from build123d import *

# Parameters (mm, degrees)
SKETCH1_W           = 70
SKETCH1_H           = 30
BOSS_EXTRUDE1_DEPTH = 10
SKETCH2_R           = 6
CUT_EXTRUDE1_DEPTH  = 6
SKETCH3_R           = 3.2
CUT_EXTRUDE2_DEPTH  = 77.393717019
SKETCH9_R           = 14.8
BOSS_EXTRUDE3_DEPTH = 6.3


with BuildPart() as part:
    # Sketch1 → Boss-Extrude1 (new body)
    with BuildSketch(Plane.XY):
        with Locations((35, -15)):
            Rectangle(SKETCH1_W, SKETCH1_H)
    extrude(amount=BOSS_EXTRUDE1_DEPTH)

    # Sketch2 → Cut-Extrude1 (cut)
    with BuildSketch(Plane.XY.offset(10)):
        with Locations((10, -15)):
            Circle(SKETCH2_R)
        with Locations((60, -15)):
            Circle(SKETCH2_R)
    extrude(amount=-CUT_EXTRUDE1_DEPTH, mode=Mode.SUBTRACT)

    # Sketch3 → Cut-Extrude2 (cut, through all)
    with BuildSketch(Plane.XY.offset(4)):
        with Locations((10, -15)):
            Circle(SKETCH3_R)
        with Locations((60, -15)):
            Circle(SKETCH3_R)
    extrude(amount=-CUT_EXTRUDE2_DEPTH, mode=Mode.SUBTRACT)

    # Sketch9 → Boss-Extrude3 (add)
    with BuildSketch(Plane(origin=(0, 0, 0), x_dir=(1, 0, 0), z_dir=(0, 1, 0))):
        with Locations((35, -25.4)):
            Circle(SKETCH9_R)
        with BuildLine():
            Line((49.8, -25.4), (49.8, -10))
            Line((49.8, -10), (20.2, -10))
            Line((20.2, -10), (20.2, -25.4))
            ThreePointArc((20.2, -25.4), (35, -10.6), (49.8, -25.4))
        make_face()
    extrude(amount=-BOSS_EXTRUDE3_DEPTH)


solid = part.part
Work out the finished part from the listing and answer in its coordinate system (mm). A direction names the side the tool comes from. Round coordinates to 2 decimals unless told otherwise and drop trailing zeros. Write each loop counter-clockwise with the first axis right and the second up, starting at its lowest first coordinate (ties: lowest second). Pieces come first, ordered by that corner, then holes. Notation, with made-up numbers: (50, 42) -> (92, 42) arc R30 ccw to (92, 67) -> close; hole circle Ø3 at (40, 60.5). An arc over 180 degrees is marked (long way). Answer as CSV lines item,"result". Start each with the question number.
(1) The part is cut by section D-D, the plane y = -10.75. Give the vertices of the cut face in (x, z), then the cut area to 3 significant figures.
(2) The mould has two halves that part along Y. Classify faces 4 (the cylindrical face through (9.22, -9.05, 7.04)), 5 (the flat face through (20.2, -3, 18)), 6 (the flat face through (35, -6.3, 25)): +Y half, -Y half, draft (parallel to the pull), parting line (faces both ways), or undercut.
(3) Each of these flat-tipped pins is pushed along its axis until it touches: pin 1 (11 mm diameter, centred on x = 60, y = -15, fed in from +Z); pin 2 (10 mm diameter, centred on x = 12, z = 30.5, fed in from -Y); pin 3 (4 mm diameter, centred on x = 52.5, y = -3.5, fed in from +Z); pin 4 (7 mm diameter, centred on y = -4.5, z = 19.5, fed in from +X). Where does it stop, or does it pass through?
(4) Find the intervals of material crossed by probe 1 along Y at (x, z) = (10, 2); probe 2 along Y at (x, z) = (10, 5.55); probe 3 along Z at (x, y) = (18, -3), in increasing order.
(5) The part is cut by section C-C, the plane z = 5. Give the vertices of the cut face in (x, y), then the cut area to 3 significant figures.
(6) A tool of negligible diameter and unlimited length cuts with its end or side. For faces 1 (the flat face through (49.8, -3, 18)), 2 (the flat face through (35, 0, 15)), 3 (the flat face through (13, -18, 4)), from which of +Z, -Z, +X, -X, +Y, -Y can it reach the whole face along a straight path? Write none if from no direction.
(7) The part is cut by section B-B, the plane y = -15. Give the vertices of the cut face in (x, z), then the cut area to 3 significant figures.
(8) The part is cut by section A-A, the plane x = 10. Give the vertices of the cut face in (y, z).
Output values:
1,outline,"(0, 0) -> (70, 0) -> (70, 10) -> (64.24, 10) -> (64.24, 4) -> (55.76, 4) -> (55.76, 10) -> (14.24, 10) -> (14.24, 4) -> (5.76, 4) -> (5.76, 10) -> (0, 10) -> close"
1,area,"598 mm²"
2,face 4,"undercut"
2,face 5,"draft"
2,face 6,"-Y half"
3,pin 1,"stops at z = 4"
3,pin 2,"passes through"
3,pin 3,"stops at z = 10"
3,pin 4,"stops at x = 49.8"
4,probe 1,"y = -30 to -18.2, -11.8 to 0"
4,probe 2,"y = -30 to -21, -9 to 0"
4,probe 3,"z = 0 to 10"
5,outline,"(0, -30) -> (70, -30) -> (70, 0) -> (0, 0) -> close; hole circle Ø12 at (10, -15); hole circle Ø12 at (60, -15)"
5,area,"1,870 mm²"
6,face 1,"+Z, +X, +Y, -Y"
6,face 2,"+Z, -Z, +X, -X, +Y"
6,face 3,"+Z"
7,outline,"(0, 0) -> (6.8, 0) -> (6.8, 4) -> (4, 4) -> (4, 10) -> (0, 10) -> close; (13.2, 0) -> (56.8, 0) -> (56.8, 4) -> (54, 4) -> (54, 10) -> (16, 10) -> (16, 4) -> (13.2, 4) -> close; (63.2, 0) -> (70, 0) -> (70, 10) -> (66, 10) -> (66, 4) -> (63.2, 4) -> close"
7,area,"505 mm²"
8,outline,"(-30, 0) -> (-18.2, 0) -> (-18.2, 4) -> (-21, 4) -> (-21, 10) -> (-30, 10) -> close; (-11.8, 0) -> (0, 0) -> (0, 10) -> (-9, 10) -> (-9, 4) -> (-11.8, 4) -> close"
